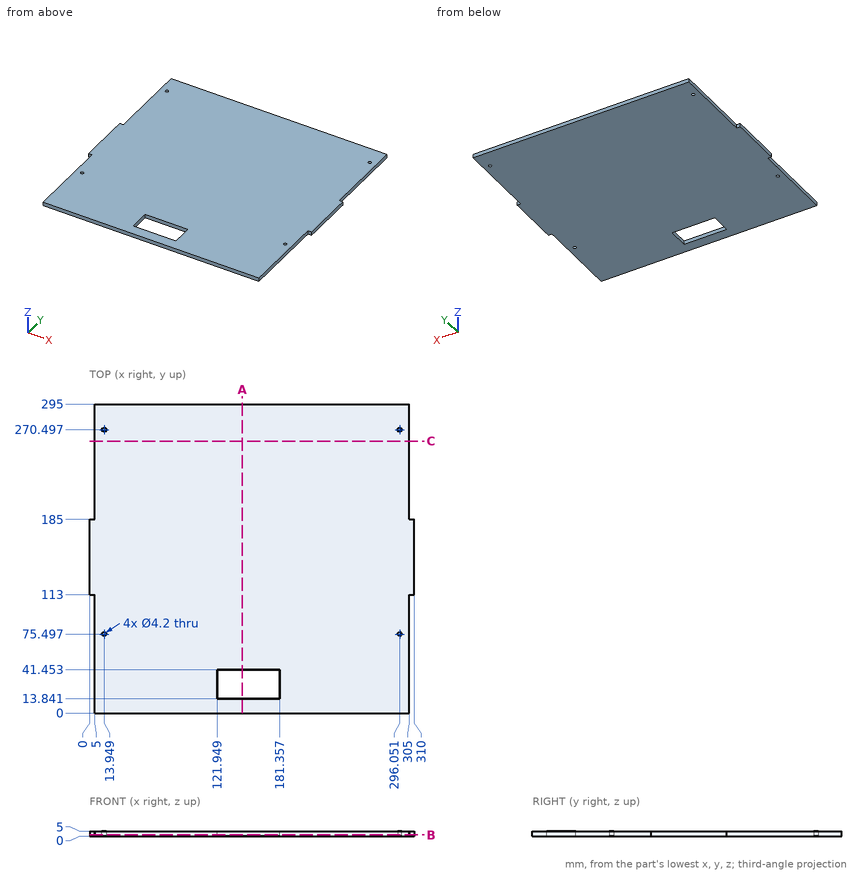
Study the drawing (mm; zero at the part's minimum x, y, z) and answer. Round coordinates to 2 decimals unless told otherwise and drop trailing zeros. Write each loop counter-clockwise with the first axis right and the second up, starting at its lowest first coordinate (ties: lowest second). Pieces come first, ordered by that corner, then holes. Notation, with made-up numbers: (6.5, 42.5) -> (15.5, 42.5) arc R33 cw to (15.5, 77.5) -> close; hole circle Ø1 at (-19, 87.5). An arc over 180 degrees is marked (long way). Write item = value, one per line.
1) Section B-B on z = 1.45 is taken. Write down the section's boundary in (x, y).
Check values:
outline = (0, 113) -> (5, 113) -> (5, 0) -> (305, 0) -> (305, 113) -> (310, 113) -> (310, 185) -> (305, 185) -> (305, 295) -> (5, 295) -> (5, 185) -> (0, 185) -> close; hole circle Ø4.2 at (13.95, 75.5); hole circle Ø4.2 at (13.95, 270.5); hole (121.95, 13.84) -> (181.36, 13.84) -> (181.36, 41.45) -> (121.95, 41.45) -> close; hole circle Ø4.2 at (296.05, 75.5); hole circle Ø4.2 at (296.05, 270.5)
2) Section A-A on x = 146 is taken. Write down the section's boundary in (y, z).
Check values:
outline = (0, 0) -> (13.84, 0) -> (13.84, 5) -> (0, 5) -> close; (41.45, 0) -> (295, 0) -> (295, 5) -> (41.45, 5) -> close
3) Straight lines are drawn through the part: line 1 along X through (y, z) = (19, 0.3); line 2 along Y through (x, z) = (144, 0.65); line 3 along X through (y, z) = (270, 1.95). For each, find the intervals that lie inside material, in ascending order. Write a range as [from, to].
Check values:
line_1 = [5, 121.95], [181.36, 305]
line_2 = [0, 13.84], [41.45, 295]
line_3 = [5, 11.91], [15.99, 294.01], [298.09, 305]
4) Given pin 1 (8 mm diameter, centred on x = 128.5, y = 236.5, fed in from -Z); pin 2 (3.5 mm diameter, centred on x = 13.95, y = 270.5, fed in from +Z); pin 3 (1.5 mm diameter, centred on x = 3.5, z = 2.5, fed in from +Y); pin 4 (2.5 mm diameter, centred on x = 308, z = 2, fed in from -Y), each flat-ended and moving along its own axis, determine where each tip first touches the part or whether it passes through.
Check values:
pin_1 = 0
pin_2 = through
pin_3 = 185
pin_4 = 113
5) Section C-C on y = 259.5 is taken. Write down the section's boundary in (x, z), plus the area to 3 significant figures.
Check values:
outline = (5, 0) -> (305, 0) -> (305, 5) -> (5, 5) -> close
area = 1,500 mm²
